Build history of the part. All positions in model axes, mm. A direction names the side the tool comes from. Round coordinates to 2 decimals unless told otherwise and drop trailing zeros. Write each loop counter-clockwise with the first axis right and the second up, starting at its lowest first coordinate (ties: lowest second). Pieces come first, ordered by that corner, then holes. Notation, with made-up numbers: M -10.75,-28 L 41.25,-28 A11 cw 41.25,-8 Z; hole C 21.25,29 d5. An arc over 180 degrees is marked long. One line per item, written item: value. Start each with the question number.
```python
from build123d import *

# Parameters (mm, degrees)
SKETCH1_R           = 3.25
BOSS_EXTRUDE1_DEPTH = 1


with BuildPart() as part:
    # Sketch1 → Boss-Extrude1 (new body)
    with BuildSketch(Plane.XY):
        with BuildLine():
            Line((-77.503167437, 240.042852563), (-77.503167437, 243.984122493))
            Line((-77.503167437, 243.984122493), (-78.99040148, 246.945192005))
            ThreePointArc((-78.99040148, 246.945192005), (-79.149249152, 247.381586959), (-79.203167437, 247.842852563))
            Line((-79.203167437, 247.842852563), (-79.203167437, 249.187318466))
            ThreePointArc((-79.203167437, 249.187318466), (-79.496060656, 249.894425247), (-80.203167437, 250.187318466))
            Line((-80.203167437, 250.187318466), (-95.103167437, 250.187318466))
            ThreePointArc((-95.103167437, 250.187318466), (-96.517380999, 250.773104903), (-97.103167437, 252.187318466))
            Line((-97.103167437, 252.187318466), (-97.103167437, 256.987318466))
            ThreePointArc((-97.103167437, 256.987318466), (-97.396060656, 257.694425247), (-98.103167437, 257.987318466))
            Line((-98.103167437, 257.987318466), (-114.103167437, 257.987318466))
            ThreePointArc((-114.103167437, 257.987318466), (-114.810274218, 257.694425247), (-115.103167437, 256.987318466))
            Line((-115.103167437, 256.987318466), (-115.103167437, 243.19838666))
            ThreePointArc((-115.103167437, 243.19838666), (-115.035769581, 242.621804655), (-114.83720999, 242.076310963))
            Line((-114.83720999, 242.076310963), (-111.767849876, 235.965242768))
            ThreePointArc((-111.767849876, 235.965242768), (-110.846211749, 234.959503948), (-109.533807323, 234.587318466))
            Line((-109.533807323, 234.587318466), (-85.503167437, 234.587318466))
            ThreePointArc((-85.503167437, 234.587318466), (-84.796060656, 234.294425247), (-84.503167437, 233.587318466))
            Line((-84.503167437, 233.587318466), (-84.503167437, 231.787318466))
            Line((-84.503167437, 231.787318466), (-83.303167437, 231.787318466))
            ThreePointArc((-83.303167437, 231.787318466), (-82.596060656, 231.494425247), (-82.303167437, 230.787318466))
            Line((-82.303167437, 230.787318466), (-82.303167437, 226.787318466))
            ThreePointArc((-82.303167437, 226.787318466), (-82.010274218, 226.080211684), (-81.303167437, 225.787318466))
            Line((-81.303167437, 225.787318466), (-78.7, 225.787318466))
            Line((-78.7, 225.787318466), (-78.7, 238.236297682))
            Line((-78.7, 238.236297682), (-77.125227291, 238.236297682))
            Line((-77.125227291, 238.236297682), (-77.125227291, 238.863736239))
            Line((-77.125227291, 238.863736239), (-77.311678075, 239.234958061))
            ThreePointArc((-77.311678075, 239.234958061), (-77.454640981, 239.627713519), (-77.503167437, 240.042852563))
        make_face()
        with Locations((-107.903167437, 240.687318466)):
            Circle(SKETCH1_R, mode=Mode.SUBTRACT)
        with Locations((-86.403167437, 244.887318466)):
            Circle(SKETCH1_R, mode=Mode.SUBTRACT)
        with Locations((-106.303167437, 252.487318466)):
            Circle(SKETCH1_R, mode=Mode.SUBTRACT)
    extrude(amount=BOSS_EXTRUDE1_DEPTH)


solid = part.part
```
Item 1: Drill centre lines: line 1 (X direction, y = 243, z = 0.15); line 2 (X direction, y = 242, z = 0.85); line 3 (Y direction, x = -85, z = 0.1). Where is each one in solid material? Low to high.
Item 2: Two-plate mould, pull along Y, no slides. Class faces 6 (the cylindrical face through (-108.608, 237.515, 0.493)), 7 (the cylindrical face through (-115.038, 242.63, 0.493)), 8 (the flat face through (-79.203, 248.5, 0.5)), 9 (the flat face through (-106, 257.987, 0.5)): pulls with the +Y half, pulls with the -Y half, needs draft (parallel to the pull), parting line crosses it, or undercut.
Item 3: Cut at A-A, the plane x = -84. Write the cut outline in (y, z), plus the area to 3 significant figures.
Item 4: Cut at C-C, the plane z = 0.15. Count the separate pieces of the cut face and the enclosed holes in it, plus the area to 3 significant figures.
Item 5: Cut at D-D, the plane x = -99.5. Write the cut outline in (y, z), plus the area to 3 significant figures.
Item 6: Cut at B-B, the plane y = 246. Write the cut outline in (x, z).
Item 7: Drop flat-ended pins along their axis: pin 1 (0.5 mm diameter, centred on y = 228, z = 0.5, fed in from -X); pin 2 (0.5 mm diameter, centred on x = -85, z = 0.5, fed in from +Y); pin 3 (0.5 mm diameter, centred on y = 254, z = 0.5, fed in from +X). Give the stop position or say it passes through.
Item 8: Which spindle directions (+Z, -Z, +X, -X, +Y, -Y) get a long thin tool onto all of the face, cutting with end or side? Do faces 1 (the flat face through (-82.303, 228.8, 0.5)), 2 (the flat face through (-87.5, 250.187, 0.5)), 3 (the cylindrical face through (-114.802, 257.702, 0.493)), 4 (the flat face through (-77.9, 238.236, 0.5)), 5 (the flat face through (-96, 242, 0)). Say none if no direction does.
Computed values:
1. line 1: x = -115.1 to -110.19, -105.62 to -89.05, -83.76 to -77.5
1. line 2: x = -114.8 to -110.88, -104.93 to -87.9, -84.91 to -77.5
1. line 3: y = 234.45 to 241.96, 247.82 to 250.19
2. face 6: undercut
2. face 7: pulls with the -Y half
2. face 8: needs draft
2. face 9: pulls with the +Y half
3. outline: M 231.79,0 L 242.7,0 L 242.7,1 L 231.79,1 Z; M 247.08,0 L 250.19,0 L 250.19,1 L 247.08,1 Z
3. area: 14.0 mm2
4. separate pieces: 1
4. enclosed holes: 3
4. area: 638 mm2
5. outline: M 234.59,0 L 257.99,0 L 257.99,1 L 234.59,1 Z
5. area: 23.4 mm2
6. outline: M -115.1,0 L -89.46,0 L -89.46,1 L -115.1,1 Z; M -83.35,0 L -78.52,0 L -78.52,1 L -83.35,1 Z
7. pin 1: stops at x = -82.3
7. pin 2: stops at y = 250.19
7. pin 3: stops at x = -97.1
8. face 1: +Z, -Z, -X, -Y
8. face 2: +Z, -Z, +X, +Y
8. face 3: +Z, -Z, -X, +Y
8. face 4: +Z, -Z, +X, -Y
8. face 5: -Z, +X, -X, +Y, -Y
